Autodesk Inventor part; units mm, degrees
ref_plane "YZ Plane" through (0, 0, 0) normal (1, 0, 0) x (0, 1, 0)
ref_plane "XZ Plane" through (0, 0, 0) normal (0, 1, 0) x (-1, 0, 0)
ref_plane "XY Plane" through (0, 0, 0) normal (0, 0, 1) x (1, 0, 0)
sketch "Skizze1" plane through (0, 0, 0) normal (0, 0, 1) x (1, 0, 0)
  line L0 (-6, 18) -> (6, 18)
  line L1 (6, 18) -> (6, 0)
  line L2 (6, 0) -> (-6, 0)
  line L3 (-6, 0) -> (-6, 18)
  point P0 (0, 0)
  point P1 (0, 0)
  dimension "d0" = 12
  dimension "d1" = 18
extrude "Extrusion1" add sketch "Skizze1" along normal blind 1
sketch "Skizze2" plane through (0, 0, 1) normal (0, 0, 1) x (1, 0, 0)
  line L0 (-4.85, 0) -> (-3.95, 0)
  line L1 (-3.95, 0) -> (-3.95, 1.5)
  line L2 (-3.95, 1.5) -> (-4.85, 1.5)
  line L3 (-4.85, 1.5) -> (-4.85, 0)
  line L4 (-4.4, 1.5) -> (-4.4, 0) construction
  line L5 (-6, 18) -> (-6, 0) construction
  circle A0 centre (-4.4, 0.9) radius 0.35 construction
  circle A1 centre (-4.4, 0) radius 0.35 construction
  point P0 (0, 0)
  dimension "d4" = 1.6
  dimension "d5" = 0.9
  dimension "d6" = 0.7
  dimension "d7" = 0.9
  dimension "d8" = 1.5
extrude "Extrusion2" cut sketch "Skizze2" against normal blind 0.05
hole "Bohrung1" at (-4.4, 0.9, 1) at (-4.4, 0, 1) direction (0, 0, -1) diameter 0.7 end through all
pattern_linear "Rechteckige Anordnung1" count 8 spacing 1.27 along (1, 0, 0) of "Extrusion2", "Bohrung1"
sketch "Skizze3" plane through (0, 0, 1) normal (0, 0, 1) x (1, 0, 0)
  line L0 (-5.8, 10) -> (-5.8, 17.8)
  line L1 (-5.8, 17.8) -> (-4, 17.8)
  line L2 (-4, 17.8) -> (-4, 14.15)
  line L3 (-4, 14.15) -> (-3.4, 14.15)
  line L4 (-3.4, 14.15) -> (-3.4, 17.8)
  line L5 (-3.4, 17.8) -> (-1.6, 17.8)
  line L6 (-1.6, 17.8) -> (-1.6, 14.15)
  line L7 (-1.6, 14.15) -> (-1, 14.15)
  line L8 (-1, 14.15) -> (-1, 17.8)
  line L9 (-1, 17.8) -> (0.8, 17.8)
  line L10 (0.8, 17.8) -> (0.8, 14.15)
  line L11 (0.8, 14.15) -> (1.4, 14.15)
  line L12 (1.4, 14.15) -> (1.4, 17.8)
  line L13 (1.4, 17.8) -> (5.8, 17.8)
  line L14 (5.8, 17.8) -> (5.8, 17.2)
  line L15 (5.8, 17.2) -> (2, 17.2)
  line L16 (2, 17.2) -> (2, 13.55)
  line L17 (2, 13.55) -> (0.2, 13.55)
  line L18 (0.2, 13.55) -> (0.2, 17.2)
  line L19 (0.2, 17.2) -> (-0.4, 17.2)
  line L20 (-0.4, 17.2) -> (-0.4, 13.55)
  line L21 (-0.4, 13.55) -> (-2.2, 13.55)
  line L22 (-2.2, 13.55) -> (-2.2, 17.2)
  line L23 (-2.2, 17.2) -> (-2.8, 17.2)
  line L24 (-2.8, 17.2) -> (-2.8, 13.55)
  line L25 (-2.8, 13.55) -> (-4.6, 13.55)
  line L26 (-4.6, 13.55) -> (-4.6, 17.2)
  line L27 (-4.6, 17.2) -> (-5.2, 17.2)
  line L28 (-5.2, 17.2) -> (-5.2, 11.8)
  line L29 (-5.2, 11.8) -> (1.4, 11.8)
  line L30 (1.4, 11.8) -> (1.4, 11.2)
  line L31 (1.4, 11.2) -> (-5.2, 11.2)
  line L32 (-5.2, 11.2) -> (-5.2, 10)
  line L33 (-5.2, 10) -> (-5.8, 10)
  line L34 (-6, 18) -> (-6, 0)
  line L35 (6, 0) -> (6, 18)
  point P0 (0, 0)
  point P1 (1.4, 11.5)
  dimension "d21" = 0.2
  dimension "d22" = 0.2
  dimension "d23" = 0.2
  dimension "d24" = 11.5
  dimension "d25" = 0.6
  dimension "d26" = 0.6
  dimension "d27" = 0.6
  dimension "d28" = 0.6
  dimension "d29" = 0.6
  dimension "d30" = 0.6
  dimension "d31" = 4.25
  dimension "d32" = 0
  dimension "d33" = 10
extrude "Extrusion3" add sketch "Skizze3" along normal blind 0.05
sketch "Skizze4" plane through (0, 0, 1) normal (0, 0, 1) x (1, 0, 0)
  line L0 (-3.5, 7) -> (0.5, 7)
  line L1 (0.5, 7) -> (0.5, 3)
  line L2 (0.5, 3) -> (-3.5, 3)
  line L3 (-3.5, 3) -> (-3.5, 7)
  line L4 (-6, 18) -> (-6, 0)
  point P0 (0, 0)
  dimension "d36" = 3
  dimension "d37" = 2.5
  dimension "d38" = 4
  dimension "d39" = 4
extrude "Extrusion4" add sketch "Skizze4" along normal blind 1.27
sketch "Skizze5" plane through (0, 0, 1) normal (0, 0, 1) x (1, 0, 0)
  line L0 (5, 7) -> (2.5, 7)
  line L1 (2.5, 7) -> (2.5, 4)
  line L2 (2.5, 4) -> (5, 4)
  line L3 (5, 4) -> (5, 7)
  line L4 (6, 0) -> (6, 18)
  point P0 (0, 0)
  dimension "d42" = 3
  dimension "d43" = 2.5
  dimension "d44" = 4
  dimension "d45" = 1
extrude "Extrusion5" add sketch "Skizze5" along normal blind 1.27
equation "\"d11\" = d6"
equation "\"d22\" = d21"
equation "\"d23\" = d21"
equation "\"d26\" = d25"
equation "\"d27\" = d25"
equation "\"d28\" = d25"
equation "\"d29\" = d27"
equation "\"d30\" = d29"
properties part number "nRF24L01+_SMD"
Source: CAD feature listing. Evaluate the final solid. Frame: model axes, mm. A direction names the side the tool comes from. Give positions to 0.01 mm unless a question says otherwise; leave off trailing zeros. Write each loop counter-clockwise with the first axis right and the second up, starting at its lowest first coordinate (ties: lowest second). Pieces come first, ordered by that corner, then holes. Notation, with made-up numbers: M 40.25,13 L 74.25,13 A16 ccw 74.25,39 Z; hole C 21.25,87 d7. An arc over 180 degrees is marked long. Return JSON: item names as keys, results as strings. Group by question number.
1) Set-up query: faces 4 (the face through (-2, 15, 1.05)), 5 (the face through (-2, 5, 2.27)). Return all of +Z, -Z, +X, -X, +Y, -Y with unobstructed straight access to the full face (end or side cutting, diameter ignored); none if empty.
2) Cut plane D-D, the plane x = -4.4. Output: boundary loops of the cut face in (y, z), then the cut area to 3 significant figures.
3) Cut plane B-B, the plane x = -1.86. Output: boundary loops of the cut face in (y, z).
4) Ray query, L1, parallel to X at y = 6.5, z = 1.1; L2, parallel to Y at x = 4.49, z = 0.35; L3, parallel to Y at x = -1, z = 1.7. Return the intervals inside material, ascending.
5) Cut plane A-A, the plane z = 1.5. Output: boundary loops of the cut face in (x, y).
6) First-contact query: pin 1 Ø1.5 at (x, y) = (4, 8.5) entering from +Z. Flat tip, straight axial feed; report the tip coordinate or a pass-through.
7) Cut plane C-C, the plane y = 11. Output: boundary loops of the cut face in (x, z).
8) Draft query along X for faces 1 (the face through (-3.5, 5, 2)), 2 (the face through (2.5, 6, 2)), 3 (the face through (0, 9, 0)). Return one class per face: released by +X, released by -X, zero draft, split by the parting line, or undercut.
Data:
{
 "1": {"face 4": "+Z, +X, -X, +Y", "face 5": "+Z, +X, -X, +Y, -Y"},
 "2": {"outline": "M 0.35,0 L 0.55,0 L 0.55,0.95 L 0.35,0.95 Z; M 1.25,0 L 18,0 L 18,1 L 17.8,1 L 17.8,1.05 L 13.55,1.05 L 13.55,1 L 11.8,1 L 11.8,1.05 L 11.2,1.05 L 11.2,1 L 1.5,1 L 1.5,0.95 L 1.25,0.95 Z", "area": "17.2 mm²"},
 "3": {"outline": "M 0.35,0 L 0.55,0 L 0.55,0.95 L 0.35,0.95 Z; M 1.25,0 L 18,0 L 18,1 L 17.8,1 L 17.8,1.05 L 13.55,1.05 L 13.55,1 L 11.8,1 L 11.8,1.05 L 11.2,1.05 L 11.2,1 L 7,1 L 7,2.27 L 3,2.27 L 3,1 L 1.5,1 L 1.5,0.95 L 1.25,0.95 Z"},
 "4": {"L1": "x = -3.5 to 0.5, 2.5 to 5", "L2": "y = 0.35 to 0.55, 1.25 to 18", "L3": "y = 3 to 7"},
 "5": {"outline": "M -3.5,3 L 0.5,3 L 0.5,7 L -3.5,7 Z; M 2.5,4 L 5,4 L 5,7 L 2.5,7 Z"},
 "6": {"pin 1": "stops at z = 1"},
 "7": {"outline": "M -6,0 L 6,0 L 6,1 L -5.2,1 L -5.2,1.05 L -5.8,1.05 L -5.8,1 L -6,1 Z"},
 "8": {"face 1": "released by -X", "face 2": "undercut", "face 3": "zero draft"}
}
